Read the model definition and answer for the solid it produces. Units are mm, in the model's axes. A direction names the side the tool comes from. Coordinates: 2 decimals unless noted, no trailing zeros. Loops run counter-clockwise (first coordinate to the right, second up) from the corner with the lowest first, then second, coordinate; pieces in that order, holes last. Notation, with made-up numbers: (55.5, 57) - (102.5, 57) arc R27 ccw to (102.5, 91) - close; hole circle Ø7 at (-36.75, 49.25). An arc over 180 degrees is marked (long way). Use one line per item in the form item = value.
from build123d import *

# Parameters (mm, degrees)
SKETCH_2_W      = 16
SKETCH_2_H      = 18
EXTRUDE_1_DEPTH = 4
EXTRUDE_START   = 3
SKETCH_3_R      = 4
EXTRUDE_3_DEPTH = 6
EXTRUDE_START_2 = 2
SKETCH_4_W      = 4
SKETCH_4_H      = 9
EXTRUDE_4_DEPTH = 1


with BuildPart() as part:
    # 草图1 → 旋转1 (revolve)
    with BuildSketch(Plane.XY, mode=Mode.PRIVATE) as revolve_1_sk:
        Polygon((8, 70), (0, 70), (0, -16), (5, -16), (7, -2), (6.5, -2), (6.5, 0), (8, 0), align=None)
    revolve(revolve_1_sk.sketch.rotate(Axis((0, 70, 0), (0, -1, 0)), 180), axis=Axis((0, 70, 0), (0, -1, 0)))

    # 草图2 → 凸台-拉伸1 (add)
    with BuildSketch(Plane(origin=(0, 70, 0), x_dir=(1, 0, 0), z_dir=(0, 1, 0))):
        Rectangle(SKETCH_2_W, SKETCH_2_H)
    extrude(amount=EXTRUDE_1_DEPTH)

    # 草图3 → 凸台-拉伸3 (add)
    with BuildSketch(Plane.XY.offset(EXTRUDE_START)):
        with BuildLine():
            Line((-8, 74), (-8, 86))
            ThreePointArc((-8, 86), (0, 94), (8, 86))
            Line((8, 86), (8, 74))
            Line((8, 74), (-8, 74))
        make_face()
        with Locations((0, 86)):
            Circle(SKETCH_3_R, mode=Mode.SUBTRACT)
    extrude_3 = extrude(amount=EXTRUDE_3_DEPTH)

    # 镜向1: 凸台-拉伸3 across plane
    add(extrude_3.mirror(Plane.XY))

    # 草图4 → 凸台-拉伸4 (add)
    with BuildSketch(Plane.XY.offset(EXTRUDE_START_2)):
        with Locations((0, -20.5)):
            Rectangle(SKETCH_4_W, SKETCH_4_H)
    extrude_4 = extrude(amount=EXTRUDE_4_DEPTH)

    # 镜向2: 凸台-拉伸4 across plane
    add(extrude_4.mirror(Plane.XY))


solid = part.part
Item 1: For a pull along X with two mould halves and no side action, classify faces 6 (the flat face through (0.6, 70, -8.2)), 7 (the flat face through (8, 78, 4)), 8 (the cylindrical face through (-0.867, 82.095, -5.958)), 9 (the cylindrical face through (0, 94, -6)) as +X half, -X half, draft (parallel to the pull), parting line (faces both ways), or undercut.
Results below:
face_6 = draft
face_7 = +X half
face_8 = undercut
face_9 = parting line
Item 2: The part is cut by section A-A on y = 79. Give the vertices of the cut face in (x, z).
Results below:
outline = (-8, -9) - (8, -9) - (8, -3) - (-8, -3) - close; (-8, 3) - (8, 3) - (8, 9) - (-8, 9) - close
Item 3: The part is cut by section C-C on y = -5.5. Give the vertices of the cut face in (x, z), plus the area to 3 significant figures.
Results below:
outline = circle Ø13 at (0, 0)
area = 133 mm²
Item 4: Which of the six approach directions +Z, -Z, +X, -X, +Y, -Y give full straight-line access (tool end or side, diameter ignored) to faces 1 (the cylindrical face through (0, 94, 6)), 2 (the flat face through (2, 82, -3)), 3 (the flat face through (0, -20, -2)), 4 (the cylindrical face through (5.158, -0.986, 3.955)), 5 (the flat face through (0, -20, 3))?
Results below:
face_1 = +Z, -Z, +Y
face_2 = +X, -X, +Y
face_3 = +X, -X, -Y
face_4 = none
face_5 = +Z, +X, -X, -Y
Item 5: Each of these flat-tipped pins is pushed along its axis until it touches: P1, Ø5, axis at y = 56.5, z = 5, coming from the -X side; P2, Ø7, axis at x = -1.5, z = 2.5, coming from the +Y side; P3, Ø1.5, axis at x = -2, y = 6, coming from the -Z side; P4, Ø4.5, axis at x = -0.5, y = -22.5, coming from the +Z side. Where does it stop, or does it pass through?
Results below:
P1 = -7.6
P2 = 94
P3 = -7.9
P4 = 3
Item 6: Find the intervals of material crossed by L1, parallel to Z at x = -4.5, y = 79; L2, parallel to Y at x = 0, z = -7.25; L3, parallel to Z at x = 0.5, y = -18, in increasing order.
Results below:
L1 = -9 to -3, 3 to 9
L2 = 0 to 82, 90 to 94
L3 = -3 to -2, 2 to 3
Item 7: The part is cut by section D-D on y = 61.5. Give the vertices of the cut face in (x, z).
Results below:
outline = circle Ø16 at (0, 0)
Item 8: The part is cut by section B-B on x = 0. Count the separate pieces of the cut face and the enclosed holes in it, plus the area to 3 significant figures.
Results below:
separate_pieces = 3
enclosed_holes = 0
area = 1,550 mm²
